Could you check a few things on this drawing? It's one solid part, dimensions in mm from its lowest x, y, z. A direction names the side the tool comes from. Coordinates: 2 decimals unless noted, no trailing zeros. Order: outer loops, then holes, each group sorted by start corner. A loop starts at its lowest first (then second) coordinate and runs counter-clockwise, first axis right, second up.
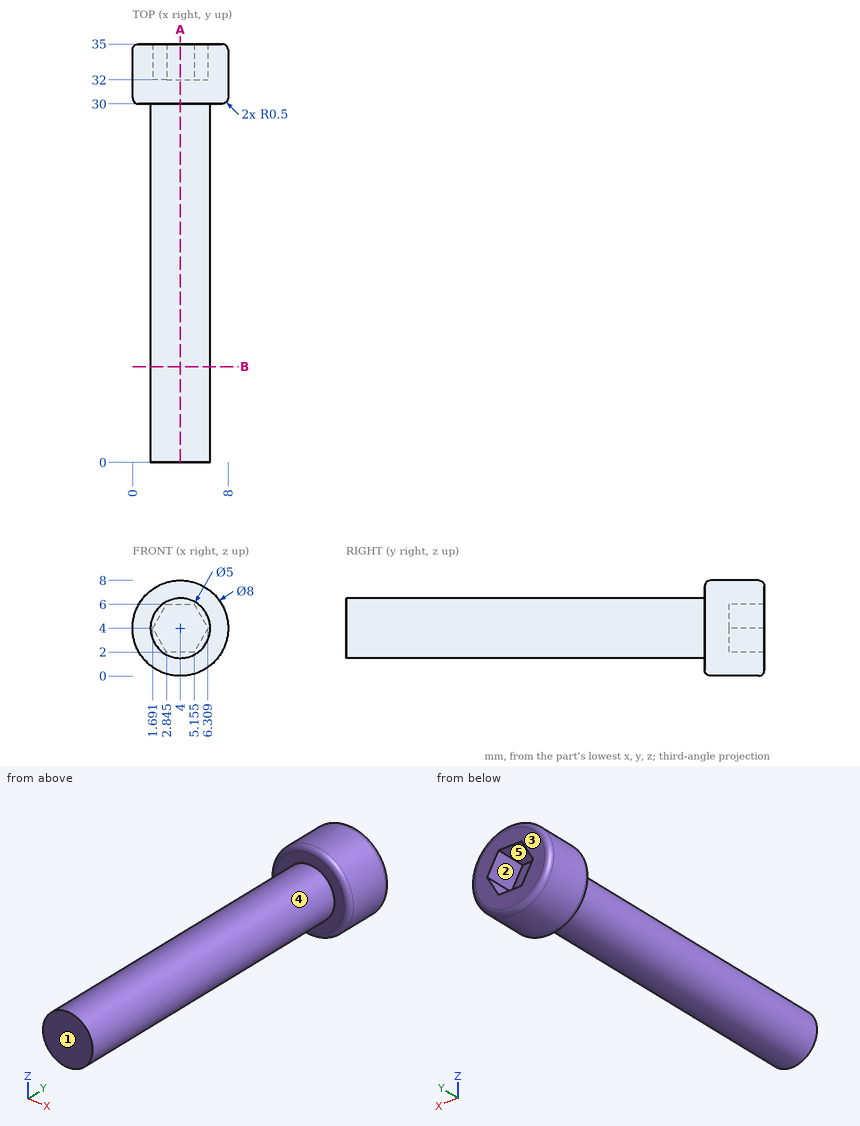
1. I'm going to push flat-ended pins straight in: pin 1 (4 mm diameter, centred on x = 1.5, y = 17, fed in from -Z); pin 2 (2 mm diameter, centred on x = 3.5, z = 4.5, fed in from +Y); pin 3 (4 mm diameter, centred on x = 1.5, y = 11, fed in from +Z). Where does each tip first touch, or does it pass through?
Completed:
pin 1: stops at z = 1.55
pin 2: stops at y = 32
pin 3: stops at z = 6.45
2. Please list where these lines run through material, in increasing order: probe 1 along X at (y, z) = (5, 2.5); probe 2 along Y at (x, z) = (0.75, 4.5); probe 3 along X at (y, z) = (32.5, 3.75) (1 decimal).
Completed:
probe 1: x = 2 to 6
probe 2: y = 30 to 35
probe 3: x = 0 to 1.8, 6.2 to 8
3. Thinking about a two-plate mould opening in Z: for the marked faces 3, 4 and 5, which applies, pulls with the +Z half, pulls with the -Z half, needs draft (parallel to the pull), parting line crosses it, or undercut?
Completed:
face 3: needs draft
face 4: parting line crosses it
face 5: undercut
4. Imagine slicing it at A-A on x = 4. Please give me the cut outline in (y, z), then the cut area to 3 significant figures.
Completed:
outline: (0, 1.5) - (30, 1.5) - (30, 0.5) arc R0.5 ccw to (30.5, 0) - (34.5, 0) arc R0.5 ccw to (35, 0.5) - (35, 2) - (32, 2) - (32, 6) - (35, 6) - (35, 7.5) arc R0.5 ccw to (34.5, 8) - (30.5, 8) arc R0.5 ccw to (30, 7.5) - (30, 6.5) - (0, 6.5) - close
area: 178 mm2
5. Imagine slicing it at B-B on y = 8. Please give me the cut outline in (x, z).
Completed:
outline: circle Ø5 at (4, 4)
6. On a 3-axis mill with a long thin cutter (end or side, diameter ignored), from which of +Z, -Z, +X, -X, +Y, -Y can I reach the whole of each face in a straight line? I mean the marked faces 1 and 2. Say none if no direction works.
Completed:
face 1: +Z, -Z, +X, -X, -Y
face 2: +Y
